Study the drawing (mm; zero at the part's minimum x, y, z) and answer. A direction names the side the tool comes from. Round coordinates to 2 decimals unless told otherwise and drop trailing zeros. Write each loop counter-clockwise with the first axis right and the second up, starting at its lowest first coordinate (ties: lowest second). Pieces come first, ordered by that corner, then holes.
(1) A cutting plane is placed at A-A, the plane x = 4.5. Give the vertices of the cut face in (y, z).
(2) Each of these flat-tipped pins is pushed along its axis until it touches: pin 1 Ø1.5 at (y, z) = (2.5, 6.5) entering from +X; pin 2 Ø1.5 at (x, y) = (19, 4) entering from -Z. Where does it stop, or does it pass through?
(3) A cutting plane is placed at B-B, the plane z = 6.5. Give the vertices of the cut face in (x, y) (1 decimal).
(4) For the marked faces 1 and 2, determine the directions among +Z, -Z, +X, -X, +Y, -Y from which every point of the face is accessible in a straight line to the end or side of a thin tool.
(5) Find the intervals of material crossed by probe 1 along X at (y, z) = (12, 8); probe 2 along Y at (x, z) = (21.5, 6.75); probe 3 along Z at (x, y) = (14, 7.5), in increasing order.
(6) A cutting plane is placed at C-C, the plane x = 25. Give the vertices of the cut face in (y, z).
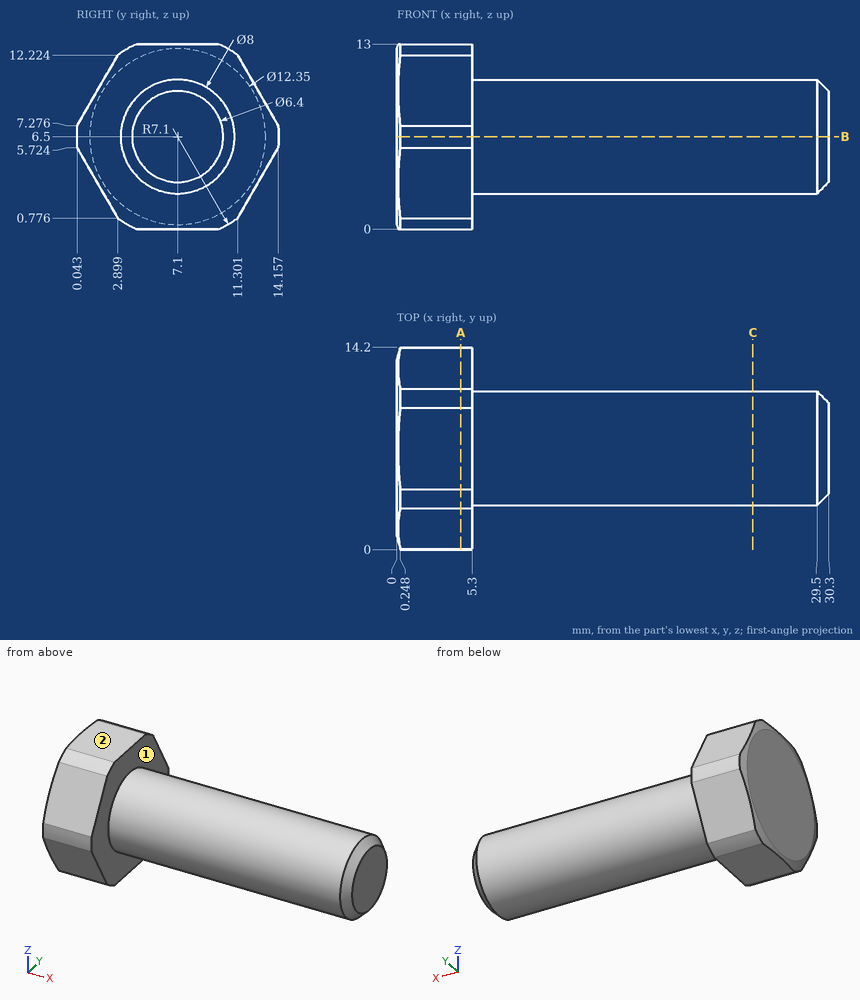
Solutions:
1. outline: (0.04, 5.72) - (2.9, 0.78) arc R7.1 ccw to (4.24, 0) - (9.96, 0) arc R7.1 ccw to (11.3, 0.78) - (14.16, 5.72) arc R7.1 ccw to (14.16, 7.28) - (11.3, 12.22) arc R7.1 ccw to (9.96, 13) - (4.24, 13) arc R7.1 ccw to (2.9, 12.22) - (0.04, 7.28) arc R7.1 ccw to start
2. pin 1: stops at x = 29.65
2. pin 2: stops at z = 3.26
3. outline: (0, 0.9) - (0.2, 0) - (5.3, 0) - (5.3, 3.1) - (29.5, 3.1) - (30.3, 3.9) - (30.3, 10.3) - (29.5, 11.1) - (5.3, 11.1) - (5.3, 14.2) - (0.2, 14.2) - (0, 13.3) - close
4. face 1: +X
4. face 2: +Z, +X, -X, +Y, -Y
5. probe 1: x = 0 to 5.3
5. probe 2: y = 3.11 to 11.09
5. probe 3: z = 2.52 to 10.48
6. outline: circle Ø8 at (7.1, 6.5)
